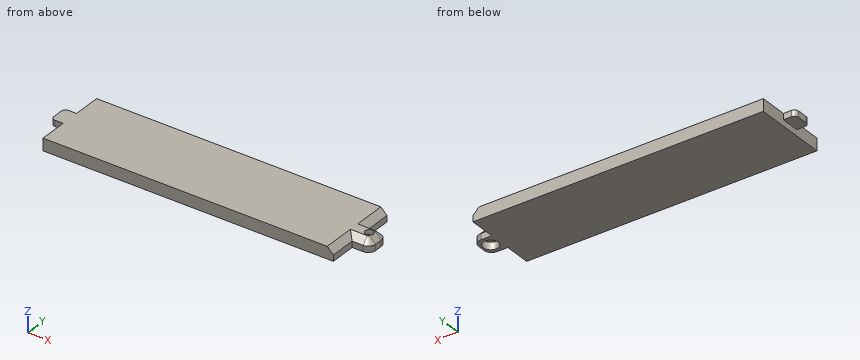
from build123d import *

# Parameters (mm, degrees)
SKETCH_1_W          = 71.6
SKETCH_1_H          = 18.4
EXTRUDE_1_DEPTH     = 3
SKETCH_3_R          = 1
EXTRUDE_2_DEPTH     = 3
SKETCH_4_R          = 1.85
CUT_EXTRUDE_1_DEPTH = 1.8
EXTRUDE_START       = -1.5
EXTRUDE_3_DEPTH     = 1.5
CHAMFER_1_SIZE      = 1.5


with BuildPart() as part:
    # 草图1 → 凸台-拉伸1 (new body)
    with BuildSketch(Plane.XY):
        Rectangle(SKETCH_1_W, SKETCH_1_H)
    extrude(amount=EXTRUDE_1_DEPTH)

    # 草图3 → 凸台-拉伸2 (add)
    with BuildSketch(Plane(origin=(0, 0, 0), x_dir=(-1, 0, 0), z_dir=(0, 0, -1))):
        with BuildLine():
            Line((-31.3, 2.75), (-38.5, 2.75))
            ThreePointArc((-38.5, 2.75), (-39.772792206, 2.222792206), (-40.3, 0.95))
            Line((-40.3, 0.95), (-40.3, -0.95))
            ThreePointArc((-40.3, -0.95), (-39.772792206, -2.222792206), (-38.5, -2.75))
            Line((-38.5, -2.75), (-31.3, -2.75))
            Line((-31.3, -2.75), (-31.3, 2.75))
        make_face()
        with Locations((-38, 0.05)):
            Circle(SKETCH_3_R, mode=Mode.SUBTRACT)
    extrude(amount=-EXTRUDE_2_DEPTH)

    # 草图4 → 切除-拉伸1 (cut)
    with BuildSketch(Plane(origin=(0, 0, 0), x_dir=(-1, 0, 0), z_dir=(0, 0, -1))):
        with Locations((-38, 0.05)):
            Circle(SKETCH_4_R)
    extrude(amount=-CUT_EXTRUDE_1_DEPTH, mode=Mode.SUBTRACT)

    # 草图5 → 凸台-拉伸3 (add)
    with BuildSketch(Plane(origin=(0, 0, 0), x_dir=(-1, 0, 0), z_dir=(0, 0, -1)).offset(EXTRUDE_START)):
        with BuildLine():
            Line((37.8, 2.3), (35.8, 2.3))
            Line((35.8, 2.3), (35.8, -2.3))
            Line((35.8, -2.3), (37.8, -2.3))
            ThreePointArc((37.8, -2.3), (38.507106781, -2.007106781), (38.8, -1.3))
            Line((38.8, -1.3), (38.8, 1.3))
            ThreePointArc((38.8, 1.3), (38.507106781, 2.007106781), (37.8, 2.3))
        make_face()
    extrude(amount=-EXTRUDE_3_DEPTH)

    # 倒角1
    # the kernel refuses this chamfer: 1.5 mm, written as the material it takes off along each edge
    with BuildSketch(Plane(origin=(35.8, 13.057524482, 3), x_dir=(0.027495876610586778, 0, -0.9996219169112968), z_dir=(0, -1, 0))) as chamfer_1_piece_1:
        Polygon((CHAMFER_1_SIZE * 0.999621916911, -CHAMFER_1_SIZE * 0.0274958766106), (-CHAMFER_1_SIZE * 0.0274958766106, -CHAMFER_1_SIZE * 0.999621916911), (0, 0), align=None)
    extrude(amount=10.307524482, mode=Mode.SUBTRACT)
    with BuildSketch(Plane(origin=(38.5, -2.75, 3), x_dir=(0, 0.9996219169112968, 0.02749587661058649), z_dir=(-1, 0, 0)), Plane(origin=(35.8, 2.75, 3), x_dir=(0, -0.9996219169112968, 0.02749587661058649), z_dir=(1, 0, 0))) as chamfer_1_piece_2:
        Polygon((CHAMFER_1_SIZE * 0.999621916911, CHAMFER_1_SIZE * 0.0274958766106), (-CHAMFER_1_SIZE * 0.0274958766106, CHAMFER_1_SIZE * 0.999621916911), (0, 0), align=None)
    extrude(amount=2.7, mode=Mode.SUBTRACT)
    with BuildSketch(Plane(origin=(38.5, -0.95, 3), x_dir=(1, 0, 0), z_dir=(0, 1, 0))) as chamfer_1_piece_3:
        Polygon((1.8 - CHAMFER_1_SIZE, 0), (1.8, CHAMFER_1_SIZE), (1.8, 0), align=None)
    revolve(axis=Axis((38.5, -0.95, 3), (0, 0, -1)), revolution_arc=90, mode=Mode.SUBTRACT)
    with BuildSketch(Plane(origin=(40.3, 0.95, 3), x_dir=(-0.9996219169112968, 0, 0.02749587661058648), z_dir=(0, -1, 0))) as chamfer_1_piece_4:
        Polygon((CHAMFER_1_SIZE * 0.999621916911, CHAMFER_1_SIZE * 0.0274958766106), (-CHAMFER_1_SIZE * 0.0274958766106, CHAMFER_1_SIZE * 0.999621916911), (0, 0), align=None)
    extrude(amount=1.9, mode=Mode.SUBTRACT)
    with BuildSketch(Plane(origin=(38.5, 0.95, 3), x_dir=(0, 1, 0), z_dir=(-1, 0, 0))) as chamfer_1_piece_5:
        Polygon((1.8 - CHAMFER_1_SIZE, 0), (1.8, CHAMFER_1_SIZE), (1.8, 0), align=None)
    revolve(axis=Axis((38.5, 0.95, 3), (0, 0, -1)), revolution_arc=90, mode=Mode.SUBTRACT)
    with BuildSketch(Plane(origin=(35.8, -2.75, 3), x_dir=(-0.9996219169112968, 0, 0.02749587661058648), z_dir=(0, -1, 0))) as chamfer_1_piece_6:
        Polygon((CHAMFER_1_SIZE * 0.999621916911, CHAMFER_1_SIZE * 0.0274958766106), (-CHAMFER_1_SIZE * 0.0274958766106, CHAMFER_1_SIZE * 0.999621916911), (0, 0), align=None)
    extrude(amount=10.307524482, mode=Mode.SUBTRACT)
    with BuildSketch(Plane(origin=(35.8, 13.057524482, 3), x_dir=(0.027495876610586778, 0, -0.9996219169112968), z_dir=(0, -1, 0))) as chamfer_1_piece_7a_section:
        Polygon((CHAMFER_1_SIZE * 0.999621916911, -CHAMFER_1_SIZE * 0.0274958766106), (-CHAMFER_1_SIZE * 0.0274958766106, -CHAMFER_1_SIZE * 0.999621916911), (0, 0), align=None)
    chamfer_1_piece_7a = extrude(amount=14.165048964, mode=Mode.PRIVATE)
    chamfer_1_piece_7a = split(chamfer_1_piece_7a, bisect_by=Plane(origin=(35.30530956, 2.75, 2.50530956), z_dir=(0, -1, 0)), keep=Keep.TOP, mode=Mode.PRIVATE)
    with BuildSketch(Plane(origin=(31.942475518, 2.75, 3), x_dir=(0, -0.9996219169112968, 0.02749587661058649), z_dir=(1, 0, 0))) as chamfer_1_piece_7b_section:
        Polygon((CHAMFER_1_SIZE * 0.999621916911, CHAMFER_1_SIZE * 0.0274958766106), (-CHAMFER_1_SIZE * 0.0274958766106, CHAMFER_1_SIZE * 0.999621916911), (0, 0), align=None)
    chamfer_1_piece_7b = extrude(amount=6.557524482, mode=Mode.PRIVATE)
    chamfer_1_piece_7b = split(chamfer_1_piece_7b, bisect_by=Plane(origin=(35.8, 2.25530956, 2.50530956), z_dir=(-1, 0, 0)), keep=Keep.TOP, mode=Mode.PRIVATE)
    chamfer_1_piece_7 = chamfer_1_piece_7a & chamfer_1_piece_7b
    add(chamfer_1_piece_7, mode=Mode.SUBTRACT)
    with BuildSketch(Plane(origin=(38.5, -2.75, 3), x_dir=(0, 0.9996219169112968, 0.02749587661058649), z_dir=(-1, 0, 0))) as chamfer_1_piece_8a_section:
        Polygon((CHAMFER_1_SIZE * 0.999621916911, CHAMFER_1_SIZE * 0.0274958766106), (-CHAMFER_1_SIZE * 0.0274958766106, CHAMFER_1_SIZE * 0.999621916911), (0, 0), align=None)
    chamfer_1_piece_8a = extrude(amount=6.557524482, mode=Mode.PRIVATE)
    chamfer_1_piece_8a = split(chamfer_1_piece_8a, bisect_by=Plane(origin=(35.8, -2.25530956, 2.50530956), z_dir=(-1, 0, 0)), keep=Keep.TOP, mode=Mode.PRIVATE)
    with BuildSketch(Plane(origin=(35.8, 1.107524482, 3), x_dir=(-0.9996219169112968, 0, 0.02749587661058648), z_dir=(0, -1, 0))) as chamfer_1_piece_8b_section:
        Polygon((CHAMFER_1_SIZE * 0.999621916911, CHAMFER_1_SIZE * 0.0274958766106), (-CHAMFER_1_SIZE * 0.0274958766106, CHAMFER_1_SIZE * 0.999621916911), (0, 0), align=None)
    chamfer_1_piece_8b = extrude(amount=14.165048964, mode=Mode.PRIVATE)
    chamfer_1_piece_8b = split(chamfer_1_piece_8b, bisect_by=Plane(origin=(35.30530956, -2.75, 2.50530956), z_dir=(0, 1, 0)), keep=Keep.TOP, mode=Mode.PRIVATE)
    chamfer_1_piece_8 = chamfer_1_piece_8a & chamfer_1_piece_8b
    add(chamfer_1_piece_8, mode=Mode.SUBTRACT)


solid = part.part
Input: part model. Units: mm. Frame: model coordinates. Give positions to 0.01 mm unless a question says otherwise; leave off trailing zeros. Write each loop counter-clockwise with the first axis right and the second up, starting at its lowest first coordinate (ties: lowest second). Pieces come first, ordered by that corner, then holes.
Q1. Section B-B, the plane y = -7.5. Output: boundary loops of the cut face in (x, z).
Q2. Section A-A, the plane z = 0.55. Output: boundary loops of the cut face in (x, y).
Q3. Material intervals for probe 1 along Y at (x, z) = (38, 1.25); probe 2 along X at (y, z) = (4, 0.2); probe 3 along X at (y, z) = (0.05, 2.4), sorted ascending.
Q4. First-contact query: P1, Ø1.2, axis at x = -36.5, z = 2.5, coming from the +Y side; P2, Ø0.5, axis at x = 37, z = 0.5, coming from the +Y side; P3, Ø0.9, axis at y = 3.5, z = 1.5, coming from the -X side. Flat tips, straight axial feed; report the tip coordinate or a pass-through.
Filled in:
1. outline: (-35.8, 0) - (35.8, 0) - (35.8, 1.5) - (34.3, 3) - (-35.8, 3) - close
2. outline: (-35.8, -9.2) - (35.8, -9.2) - (35.8, -2.75) - (38.5, -2.75) arc R1.8 ccw to (40.3, -0.95) - (40.3, 0.95) arc R1.8 ccw to (38.5, 2.75) - (35.8, 2.75) - (35.8, 9.2) - (-35.8, 9.2) - close; hole circle Ø3.7 at (38, 0.05)
3. probe 1: y = -2.75 to -1.8, 1.9 to 2.75
3. probe 2: x = -35.8 to 35.8
3. probe 3: x = -38.8 to 37, 39 to 39.4
4. P1: stops at y = 2.3
4. P2: stops at y = 2.75
4. P3: stops at x = -35.8
